```python
from build123d import *

# Parameters (mm, degrees)
SKETCH1_R           = 4.8
SKETCH1_R_2         = 1.5
BOSS_EXTRUDE3_DEPTH = 4


with BuildPart() as part:
    # Sketch1 → Boss-Extrude3 (new body)
    with BuildSketch(Plane.XY):
        Polygon((-125, -100), (150, -100), (150, 100), (-125, 100), (-150, 0), align=None)
        with BuildLine():
            Line((0, -33.333333333), (-1.592872426, -36.333333333))
            ThreePointArc((-1.592872426, -36.333333333), (-50, -81.833333333), (-98.407127574, -36.333333333))
            Line((-98.407127574, -36.333333333), (-100, -33.333333333))
            Line((-100, -33.333333333), (-98.407127574, -30.333333333))
            ThreePointArc((-98.407127574, -30.333333333), (-50, 15.166666667), (-1.592872426, -30.333333333))
            Line((-1.592872426, -30.333333333), (0, -33.333333333))
        make_face(mode=Mode.SUBTRACT)
        with Locations((107.142857143, -71.428571429)):
            Circle(SKETCH1_R, mode=Mode.SUBTRACT)
        with Locations((-107.142857143, 71.428571429)):
            Circle(SKETCH1_R, mode=Mode.SUBTRACT)
        with Locations((21.832408692, 6.152026506)):
            Circle(SKETCH1_R_2, mode=Mode.SUBTRACT)
        with Locations((37.332408692, 21.652026506)):
            Circle(SKETCH1_R, mode=Mode.SUBTRACT)
        with Locations((52.832408692, 6.152026506)):
            Circle(SKETCH1_R_2, mode=Mode.SUBTRACT)
        with Locations((21.832408692, 37.152026506)):
            Circle(SKETCH1_R_2, mode=Mode.SUBTRACT)
        with Locations((52.832408692, 37.152026506)):
            Circle(SKETCH1_R_2, mode=Mode.SUBTRACT)
        with Locations((107.142857143, 71.428571429)):
            Circle(SKETCH1_R, mode=Mode.SUBTRACT)
    extrude(amount=BOSS_EXTRUDE3_DEPTH)


solid = part.part
```
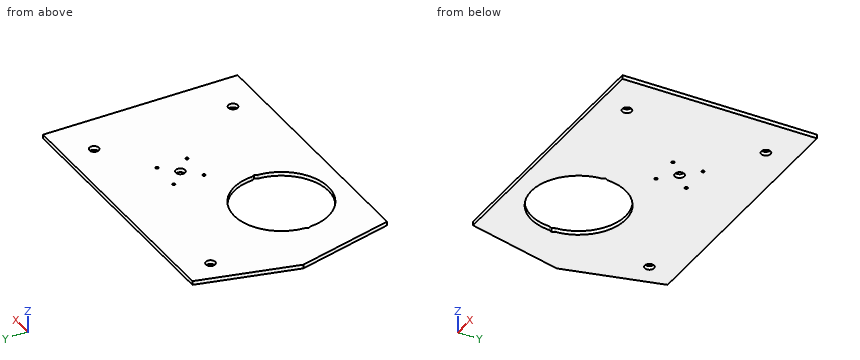
Build history of the part. All positions in model axes, mm. Give positions to 0.01 mm unless a question says otherwise; leave off trailing zeros. Order: outer loops, then holes, each group sorted by start corner. A loop starts at its lowest first (then second) coordinate and runs counter-clockwise, first axis right, second up. Notation, with made-up numbers: M -39,60.5 L -15,60.5 A33 ccw -15,93.5 Z; hole C 17.25,9.5 d3. An arc over 180 degrees is marked long. Return JSON: item names as keys, results as strings.
Q1. Wall check: probe 1 along Y at (x, z) = (37, 2); probe 2 along Y at (x, z) = (-74, 0.45); probe 3 along X at (y, z) = (22.5, 2.6) (3 decimals). Give the ranges that are in metal, low to high. Write a range as from..to.
Answer list:
{"probe 1": "y = -100..16.86, 26.44..100", "probe 2": "y = -100..-75.48, 8.81..100", "probe 3": "x = -144.375..32.608, 42.057..150"}
Q2. Band-saw the part on B-B (y = -4.5). Give the cut face in (x, z) (3 decimals).
Answer list:
{"outline": "M -148.875,0 L -88.999,0 L -88.999,4 L -148.875,4 Z; M -11.001,0 L 150,0 L 150,4 L -11.001,4 Z"}
Q3. Band-saw the part on A-A (x = -50). Give the cut face in (y, z).
Answer list:
{"outline": "M -100,0 L -81.83,0 L -81.83,4 L -100,4 Z; M 15.17,0 L 100,0 L 100,4 L 15.17,4 Z"}
Q4. Band-saw the part on D-D (y = 45.5). Give the cut face in (x, z) (3 decimals).
Answer list:
{"outline": "M -138.625,0 L 150,0 L 150,4 L -138.625,4 Z"}
Q5. Band-saw the part on C-C (z = 0.8). Count the separate pieces of the cut face and the enclosed holes in it, then the cut area to 3 significant figures.
Answer list:
{"separate pieces": "1", "enclosed holes": "9", "area": "49,800 mm^2"}
